The model under review builds one solid part; all positions refer to its coordinate system, in mm. A direction names the side the tool comes from. Give positions to 0.01 mm unless a question says otherwise; leave off trailing zeros. Order: outer loops, then holes, each group sorted by start corner. A loop starts at its lowest first (then second) coordinate and runs counter-clockwise, first axis right, second up.
```python
from build123d import *

# Parameters (mm, degrees)
F0_W      = 61.210394
F0_H      = 39.28775
F1_DEPTH  = 25.4
F2_R      = 5.08
F1_FACE_W = 56.130394
F1_FACE_H = 34.20775
F3_DEPTH  = 25.4


with BuildPart() as f1:
    # F0 (on Top) → F1 (new body)
    with BuildSketch(Plane.XY):
        with Locations((30.605197, 19.643875)):
            Rectangle(F0_W, F0_H)
    extrude(amount=F1_DEPTH)

    # F2
    f2_edges = [f1.edges().sort_by_distance(p)[0] for p in [
        (0, 0, 12.7),
        (61.210394, 0, 12.7),
        (30.605197, 0, 0),
        (30.605197, 0, 25.4),
        (61.210394, 19.643875, 25.4),
        (61.210394, 39.28775, 12.7),
        (61.210394, 19.643875, 0),
    ]]
    fillet(f2_edges, radius=F2_R)

    # F1_face (on face) → F3 (join)
    with BuildSketch(Plane(origin=(28.065197, 22.183875, 25.4), x_dir=(1, 0, 0), z_dir=(0, 0, 1))):
        Rectangle(F1_FACE_W, F1_FACE_H)
    extrude(amount=F3_DEPTH)


solid = f1.part
```
Item 1: Take a section at C-C (z = 40.5). Give the boundary of the cut face in (x, y), and give its area (3 significant figures).
Values found:
outline: (0, 5.08) - (56.13, 5.08) - (56.13, 39.29) - (0, 39.29) - close
area: 1,920 mm2
Item 2: Take a section at A-A (y = 28). Give the boundary of the cut face in (x, z), and give its area (3 significant figures).
Values found:
outline: (0, 0) - (56.13, 0) arc R5.08 ccw to (61.21, 5.08) - (61.21, 20.32) arc R5.08 ccw to (56.13, 25.4) - (56.13, 50.8) - (0, 50.8) - close
area: 2,970 mm2
Item 3: For line 1 (X direction, y = 12.5, z = 31); line 2 (Y direction, x = 30.5, z = 42); line 3 (Y direction, x = 56.5, z = 4), list the stretches that pass through material, from the lowest coordinate up.
Values found:
line 1: x = 0 to 56.13
line 2: y = 5.08 to 39.29
line 3: y = 0.13 to 39.27
Item 4: Take a section at D-D (y = 2). Give the boundary of the cut face in (x, z).
Values found:
outline: (1.04, 1.04) - (56.13, 1.04) arc R4.04 ccw to (60.17, 5.08) - (60.17, 20.32) arc R4.04 ccw to (56.13, 24.36) - (1.04, 24.36) - close
Item 5: For faces 1 (the flat face through (56.13, 22, 38)), 2 (the flat face through (28, 5.08, 38)), 3 (the flat face through (28, 22, 0)), list the 3-axis set-ups (+Z, -Z, +X, -X, +Y, -Y) from which the entire face can be reached by the end or side of a thin tool; tool diameter is ignored.
Values found:
face 1: +Z, +X, +Y, -Y
face 2: +Z, +X, -X, -Y
face 3: -Z, +X, -X, +Y, -Y
Item 6: Take a section at B-B (x = 44.5). Give the boundary of the cut face in (y, z).
Values found:
outline: (0, 5.08) arc R5.08 ccw to (5.08, 0) - (39.29, 0) - (39.29, 50.8) - (5.08, 50.8) - (5.08, 25.4) arc R5.08 ccw to (0, 20.32) - close
Item 7: Clearance check with flat-ended pins moving along their axes: pin 1 Ø12 at (x, y) = (33.5, 32.5) entering from -Z; pin 2 Ø12.5 at (y, z) = (26, 35.5) entering from +X; pin 3 Ø2 at (x, z) = (22.5, 34) entering from -Y; pin 4 Ø1.5 at (y, z) = (13, 25.5) entering from +X. State where each tip first meets the part, or that it passes through.
Values found:
pin 1: stops at z = 0
pin 2: stops at x = 56.13
pin 3: stops at y = 5.08
pin 4: stops at x = 58.62
